Geometry: final body of the model. Coordinates: model frame, mm. Give positions to 0.01 mm unless a question says otherwise; leave off trailing zeros. Loops run counter-clockwise (first coordinate to the right, second up) from the corner with the lowest first, then second, coordinate; pieces in that order, holes last. Notation, with made-up numbers: (-34.5, 54) -> (-21.5, 54) arc R13 cw to (-21.5, 65) -> close; hole circle Ø11 at (-39, 46.5). An arc over 180 degrees is marked (long way). One line per question, with ' | ' between items. Start each with the question number.
Item 1: Section A-A on y = 60. Return loops of the section in (x, z), then the cut area to 3 significant figures.
Item 2: Section B-B on z = -64. Return loops of the section in (x, y).
Item 3: Section C-C on x = 0.9. Give the number of separate pieces and of enclosed holes in the cut face, then the cut area to 3 significant figures.
Item 4: Pin query (flat end, axial travel): P1, Ø1.5, axis at x = 1.5, z = -53.5, coming from the +Y side; P2, Ø2.5, axis at y = 22, z = -8.5, coming from the -X side. Return the tip coordinate at first contact, or that it passes through.
Item 5: Material intervals for line 1 along Y through (x, z) = (1.35, -8.5); line 2 along Z through (x, y) = (2.35, 58.5); line 3 along Z through (x, y) = (1.5, 89), sorted ascending. Write a range as [from, to].
from build123d import *

# Parameters (mm, degrees)
CROQUIS1_W              = 105
CROQUIS1_H              = 170
CROQUIS1_R              = 1.5
CROQUIS1_W_2            = 3
CROQUIS1_H_2            = 32
SALIENTE_EXTRUIR1_DEPTH = 3
CROQUIS2_W              = 3
CROQUIS2_H              = 16
SALIENTE_EXTRUIR2_DEPTH = 3
CORTAR_EXTRUIR1_DEPTH   = 3


with BuildPart() as part:
    # Croquis1 → Saliente-Extruir1 (new body)
    with BuildSketch(Plane(origin=(0, 0, 0), x_dir=(0, 0, -1), z_dir=(1, 0, 0))):
        with Locations((52.5, 85)):
            Rectangle(CROQUIS1_W, CROQUIS1_H)
        with Locations((96.5, 160)):
            Circle(CROQUIS1_R, mode=Mode.SUBTRACT)
        with Locations((96.5, 22)):
            Circle(CROQUIS1_R, mode=Mode.SUBTRACT)
        with Locations((96.5, 90)):
            Circle(CROQUIS1_R, mode=Mode.SUBTRACT)
        with Locations(Location((8.5, 22, 0), (0, 0, 180))):
            Circle(CROQUIS1_R, mode=Mode.SUBTRACT)
        with Locations(Location((8.5, 90, 0), (0, 0, 180))):
            Circle(CROQUIS1_R, mode=Mode.SUBTRACT)
        with Locations(Location((8.5, 160, 0), (0, 0, 180))):
            Circle(CROQUIS1_R, mode=Mode.SUBTRACT)
        with Locations((96.5, 58)):
            Rectangle(CROQUIS1_W_2, CROQUIS1_H_2, mode=Mode.SUBTRACT)
        with Locations((96.5, 122)):
            Rectangle(CROQUIS1_W_2, CROQUIS1_H_2, mode=Mode.SUBTRACT)
        with Locations((8.5, 58)):
            Rectangle(CROQUIS1_W_2, CROQUIS1_H_2, mode=Mode.SUBTRACT)
        with Locations((8.5, 122)):
            Rectangle(CROQUIS1_W_2, CROQUIS1_H_2, mode=Mode.SUBTRACT)
    extrude(amount=SALIENTE_EXTRUIR1_DEPTH)

    # Croquis2 → Saliente-Extruir2 (add)
    with BuildSketch(Plane(origin=(0, 170, 0), x_dir=(1, 0, 0), z_dir=(0, 1, 0))):
        with Locations((1.5, 76.5)):
            Rectangle(CROQUIS2_W, CROQUIS2_H)
        with Locations((1.5, 28.5)):
            Rectangle(CROQUIS2_W, CROQUIS2_H)
    extrude(amount=SALIENTE_EXTRUIR2_DEPTH)

    # Croquis3 → Cortar-Extruir1 (cut)
    with BuildSketch(Plane.ZY):
        with BuildLine():
            Line((-11, 168), (-11, 170))
            Line((-11, 170), (-14, 170))
            Line((-14, 170), (-14, 168))
            Line((-14, 168), (-14.75, 168))
            ThreePointArc((-14.75, 168), (-15.176776695, 168.176776695), (-15, 167.75))
            Line((-15, 167.75), (-15, 165.25))
            ThreePointArc((-15, 165.25), (-15.176776695, 164.823223305), (-14.75, 165))
            Line((-14.75, 165), (-14, 165))
            Line((-14, 165), (-14, 164))
            Line((-14, 164), (-11, 164))
            Line((-11, 164), (-11, 165))
            Line((-11, 165), (-10.25, 165))
            ThreePointArc((-10.25, 165), (-9.823223305, 164.823223305), (-10, 165.25))
            Line((-10, 165.25), (-10, 167.75))
            ThreePointArc((-10, 167.75), (-9.823223305, 168.176776695), (-10.25, 168))
            Line((-10.25, 168), (-11, 168))
        make_face()
        with BuildLine():
            Line((-91, 168), (-91, 170))
            Line((-91, 170), (-94, 170))
            Line((-94, 170), (-94, 168))
            Line((-94, 168), (-94.75, 168))
            ThreePointArc((-94.75, 168), (-95.176776695, 168.176776695), (-95, 167.75))
            Line((-95, 167.75), (-95, 165.25))
            ThreePointArc((-95, 165.25), (-95.176776695, 164.823223305), (-94.75, 165))
            Line((-94.75, 165), (-94, 165))
            Line((-94, 165), (-94, 164))
            Line((-94, 164), (-91, 164))
            Line((-91, 164), (-91, 165))
            Line((-91, 165), (-90.25, 165))
            ThreePointArc((-90.25, 165), (-89.823223305, 164.823223305), (-90, 165.25))
            Line((-90, 165.25), (-90, 167.75))
            ThreePointArc((-90, 167.75), (-89.823223305, 168.176776695), (-90.25, 168))
            Line((-90.25, 168), (-91, 168))
        make_face()
    extrude(amount=-CORTAR_EXTRUIR1_DEPTH, mode=Mode.SUBTRACT)


solid = part.part
Result sheet:
1) outline: (0, -105) -> (3, -105) -> (3, -98) -> (0, -98) -> close; (0, -95) -> (3, -95) -> (3, -10) -> (0, -10) -> close; (0, -7) -> (3, -7) -> (3, 0) -> (0, 0) -> close | area: 297 mm²
2) outline: (0, 0) -> (3, 0) -> (3, 170) -> (0, 170) -> close
3) separate pieces: 1 | enclosed holes: 10 | area: 17,500 mm²
4) P1: stops at y = 170 | P2: passes through
5) line 1: y = [0, 20.5], [23.5, 42], [74, 88.5], [91.5, 106], [138, 158.5], [161.5, 170] | line 2: z = [-105, -98], [-95, -10], [-7, 0] | line 3: z = [-105, -97.62], [-95.38, -9.62], [-7.38, 0]
